Autodesk Inventor part; units mm, degrees
ref_plane "YZ Plane" through (0, 0, 0) normal (1, 0, 0) x (0, 1, 0)
ref_plane "XZ Plane" through (0, 0, 0) normal (0, 1, 0) x (-1, 0, 0)
ref_plane "XY Plane" through (0, 0, 0) normal (0, 0, 1) x (1, 0, 0)
sketch "Boceto1" plane through (0, 0, 0) normal (0, 1, 0) x (-1, 0, 0)
  line L0 (0, 0) -> (65, 0) construction
  line L1 (0, 0) -> (-65, 0) construction
  line L2 (65, 0) -> (65, 34)
  line L3 (-65, 0) -> (-65, 34)
  line L4 (65, 34) -> (57.5, 34) construction
  line L5 (-65, 34) -> (-57.5, 34) construction
  arc A0 (65, 34) -> (57.5, 41.5) centre (57.5, 34) ccw
  arc A1 (-57.5, 41.5) -> (-65, 34) centre (-57.5, 34) ccw
  line L6 (-57.5, 41.5) -> (57.5, 41.5)
  dimension "d0" = 65
  dimension "d1" = 65
  dimension "d2" = 34
  dimension "d3" = 34
  dimension "d5" = 7.5
  dimension "d6" = 7.5
sketch "Boceto2" plane through (0, 0, 0) normal (0, 0, 1) x (1, 0, 0)
  circle A0 centre (-65, 0) radius 10
  point P0 (0, 0)
  dimension "d7" = 20
sweep "Barrido1" add profiles "Boceto2" path "Boceto1"
sketch "Boceto3" plane through (65, 0, 0) normal (0, 0, -1) x (-1, 0, 0)
  circle A0 centre (0, 0) radius 2.3813
  circle A1 centre (130, 0) radius 2.3812
  point P0 (65, 0)
  dimension "d10" = 4.7625
  dimension "d11" = 4.7625
extrude "Extrusión1" cut sketch "Boceto3" against normal blind 19.05
properties part number "mango_zona_calor" material "Plástico PC/ABS"
The model under review builds one solid part; all positions refer to its coordinate system, in mm. A direction names the side the tool comes from. Give positions to 0.01 mm unless a question says otherwise; leave off trailing zeros. Write each loop counter-clockwise with the first axis right and the second up, starting at its lowest first coordinate (ties: lowest second). Pieces come first, ordered by that corner, then holes. Notation, with made-up numbers: M 27.25,54 L 38.25,54 A10 ccw 38.25,61 Z; hole C 24,42 d10. An arc over 180 degrees is marked long. One line per question, with ' | ' between items. Start each with the question number.
Item 1: Draft analysis for pull direction X (two halves, no side actions). For faces 4 (the flat face through (63, -2, 0)), 5 (the cylindrical face through (62.73, 0.72, 9.39)), state which applies: released by +X, released by -X, zero draft, split by the parting line, or undercut.
Item 2: Wall thickness on line 1 (Y direction, x = 65, z = 9); line 2 (X direction, y = -1.5, z = 4.5); line 3 (X direction, y = 8, z = 29): over which ranges is each line inside the solid? List them lowest first. Write a range as from..to.
Item 3: For faces 1 (the flat face through (-63, -2, 0)), 2 (the cylindrical face through (0.8, 0.44, 51.49)), 3 (the flat face through (65, 0, 19.05)), list the 3-axis set-ups (+Z, -Z, +X, -X, +Y, -Y) from which the entire face can be reached by the end or side of a thin tool; tool diameter is ignored.
Item 4: We need section A-A on x = -2.5. Write out the cut boundary in (y, z), plus the area to 3 significant figures.
Item 5: For pin 1 (2 mm diameter, centred on y = -7, z = 19.5, fed in from +X); pin 2 (4 mm diameter, centred on x = -64, y = -1, fed in from -Z); pin 3 (3 mm diameter, centred on y = 8, z = 33.5, fed in from +X); pin 4 (4.5 mm diameter, centred on x = 65, y = 0, fed in from +Z), all flat-tipped, find the tip position at first contact; note any pin that passes through.
Results found:
1) face 4: zero draft | face 5: undercut
2) line 1: y = -10..-2.38, 2.38..10 | line 2: x = -74.89..-66.85, -63.15..-55.11, 55.11..63.15, 66.85..74.89 | line 3: x = -71..-59, 59..71
3) face 1: -Z, +X, -X, +Y, -Y | face 2: none | face 3: -Z
4) outline: C 0,41.5 d20 | area: 314 mm2
5) pin 1: stops at x = 73 | pin 2: stops at z = 0 | pin 3: stops at x = 72.6 | pin 4: stops at z = 50.69
